from build123d import *

# Parameters (mm, degrees)
SKETCH_1_R          = 1.5
EXTRUDE_2_DEPTH     = 2
SKETCH_2_R          = 1.5
CUT_EXTRUDE_1_DEPTH = 10
SKETCH_3_R          = 0.5
CUT_EXTRUDE_2_DEPTH = 3
FILLET_1_R          = 1
SKETCH_4_R          = 0.5
SKETCH_4_W          = 24
SKETCH_4_H          = 6
CUT_EXTRUDE_3_DEPTH = 3


with BuildPart() as part:
    # 草图1 → 凸台-拉伸2 (new body)
    with BuildSketch(Plane.XY):
        with BuildLine():
            Line((56, -66.5), (44, -66.5))
            Line((44, -66.5), (44, -41.3))
            Line((44, -41.3), (56, -41.3))
            Line((56, -41.3), (56, -21.3))
            Line((56, -21.3), (44, -21.3))
            Line((44, -21.3), (44, -5.1))
            Line((44, -5.1), (56, -5.1))
            Line((56, -5.1), (56, 14.9))
            Line((56, 14.9), (44, 14.9))
            Line((44, 14.9), (44, 30.5))
            Line((44, 30.5), (56, 30.5))
            Line((56, 30.5), (56, 50.5))
            Line((56, 50.5), (44, 50.5))
            Line((44, 50.5), (44, 74.5))
            Line((44, 74.5), (0, 74.5))
            ThreePointArc((0, 74.5), (-23.145322016, 70.813445537), (-44, 60.118632719))
            Line((-44, 60.118632719), (-44, 40.5))
            Line((-44, 40.5), (-52, 40.5))
            Line((-52, 40.5), (-52, 20.5))
            Line((-52, 20.5), (-44, 20.5))
            Line((-44, 20.5), (-44, 0.5))
            Line((-44, 0.5), (-52, 0.5))
            Line((-52, 0.5), (-52, -19.5))
            Line((-52, -19.5), (-44, -19.5))
            Line((-44, -19.5), (-44, -44.5))
            Line((-44, -44.5), (-52, -44.5))
            Line((-52, -44.5), (-52, -59.5))
            Line((-52, -59.5), (-44, -59.5))
            Line((-44, -59.5), (-44, -64.5))
            Line((-44, -64.5), (-34, -74.5))
            Line((-34, -74.5), (-24, -74.5))
            Line((-24, -74.5), (-24, -92.324700538))
            Line((-24, -92.324700538), (-14.522169318, -97.796728634))
            Line((-14.522169318, -97.796728634), (-8, -86.5))
            Line((-8, -86.5), (-8, -74.5))
            Line((-8, -74.5), (19, -74.5))
            Line((19, -74.5), (19, -86.5))
            Line((19, -86.5), (56, -86.5))
            Line((56, -86.5), (56, -66.5))
        make_face()
        with Locations((24, -81.5)):
            Circle(SKETCH_1_R, mode=Mode.SUBTRACT)
        with Locations((39, -81.5)):
            Circle(SKETCH_1_R, mode=Mode.SUBTRACT)
        with Locations((51, -81.5)):
            Circle(SKETCH_1_R, mode=Mode.SUBTRACT)
        with Locations((16, 35.5)):
            Circle(SKETCH_1_R, mode=Mode.SUBTRACT)
        with Locations((39, 69.5)):
            Circle(SKETCH_1_R, mode=Mode.SUBTRACT)
        with Locations((39, -69.5)):
            Circle(SKETCH_1_R, mode=Mode.SUBTRACT)
        with Locations((-14, 35.5)):
            Circle(SKETCH_1_R, mode=Mode.SUBTRACT)
        with Locations((-16, -81.5)):
            Circle(SKETCH_1_R, mode=Mode.SUBTRACT)
        with Locations((-16, -91.17)):
            Circle(SKETCH_1_R, mode=Mode.SUBTRACT)
        with Locations((51, -35.5)):
            Circle(SKETCH_1_R, mode=Mode.SUBTRACT)
        with Locations((51, 4.5)):
            Circle(SKETCH_1_R, mode=Mode.SUBTRACT)
        with Locations((51, 35.5)):
            Circle(SKETCH_1_R, mode=Mode.SUBTRACT)
    extrude(amount=EXTRUDE_2_DEPTH)

    # 草图2 → 切除-拉伸1 (cut)
    with BuildSketch(Plane(origin=(0, 0, 0), x_dir=(-1, 0, 0), z_dir=(0, 0, -1))):
        with Locations((48.75, 30.5)):
            Circle(SKETCH_2_R)
        with Locations((48.75, -9.5)):
            Circle(SKETCH_2_R)
        with Locations((48.75, -52)):
            Circle(SKETCH_2_R)
    extrude(amount=-CUT_EXTRUDE_1_DEPTH, mode=Mode.SUBTRACT)

    # 草图3 → 切除-拉伸2 (cut, through all)
    with BuildSketch(Plane(origin=(0, 0, 0), x_dir=(-1, 0, 0), z_dir=(0, 0, -1))):
        with Locations((-44, 50.5)):
            Circle(SKETCH_3_R)
        with Locations((-44, 30.5)):
            Circle(SKETCH_3_R)
        with Locations((-44, 14.9)):
            Circle(SKETCH_3_R)
        with Locations((-44, -5.1)):
            Circle(SKETCH_3_R)
        with Locations((-44, -21.3)):
            Circle(SKETCH_3_R)
        with Locations((-44, -41.3)):
            Circle(SKETCH_3_R)
        with Locations((-44, -66.5)):
            Circle(SKETCH_3_R)
        with Locations((44, 40.5)):
            Circle(SKETCH_3_R)
        with Locations((44, 20.5)):
            Circle(SKETCH_3_R)
        with Locations((44, 0.5)):
            Circle(SKETCH_3_R)
        with Locations((44, -19.5)):
            Circle(SKETCH_3_R)
        with Locations((44, -44.5)):
            Circle(SKETCH_3_R)
        with Locations((44, -59.5)):
            Circle(SKETCH_3_R)
        with Locations((-19, -74.5)):
            Circle(SKETCH_3_R)
        with Locations((8, -74.5)):
            Circle(SKETCH_3_R)
        with Locations((24, -74.5)):
            Circle(SKETCH_3_R)
    extrude(amount=-CUT_EXTRUDE_2_DEPTH, mode=Mode.SUBTRACT)

    # 圆角1
    fillet_1_edges = [part.edges().sort_by_distance(p)[0] for p in [
        (-8, -86.5, 1),
        (-14.522169318, -97.796728634, 1),
        (-24, -92.324700538, 1),
        (-34, -74.5, 1),
        (-44, -64.5, 1),
        (-52, -59.5, 1),
        (-52, -44.5, 1),
        (-52, -19.5, 1),
        (-52, 0.5, 1),
        (-52, 20.5, 1),
        (-52, 40.5, 1),
        (-44, 60.118632719, 1),
        (44, 74.5, 1),
        (56, 50.5, 1),
        (56, 30.5, 1),
        (56, -5.1, 1),
        (56, -21.3, 1),
        (56, -41.3, 1),
        (56, -66.5, 1),
        (56, -86.5, 1),
        (19, -86.5, 1),
    ]]
    fillet(fillet_1_edges, radius=FILLET_1_R)

    # 草图4 → 切除-拉伸3 (cut, through all)
    with BuildSketch(Plane(origin=(0, 0, 0), x_dir=(-1, 0, 0), z_dir=(0, 0, -1))):
        with BuildLine():
            Line((-12, 64), (-12, 64.5))
            Line((-12, 64.5), (-11.5, 64.5))
            ThreePointArc((-11.5, 64.5), (-12.353553391, 64.853553391), (-12, 64))
        make_face()
        with BuildLine():
            Line((-11.5, 64.5), (-12, 64.5))
            Line((-12, 64.5), (-12, 64))
            ThreePointArc((-12, 64), (-11.646446609, 64.146446609), (-11.5, 64.5))
        make_face()
        with BuildLine():
            ThreePointArc((-11.5, 58.5), (-11.646446609, 58.853553391), (-12, 59))
            Line((-12, 59), (-12, 58.5))
            Line((-12, 58.5), (-11.5, 58.5))
        make_face()
        with BuildLine():
            Line((-12, 58.5), (-12, 59))
            ThreePointArc((-12, 59), (-12.353553391, 58.146446609), (-11.5, 58.5))
            Line((-11.5, 58.5), (-12, 58.5))
        make_face()
        with Locations((12, 58.5)):
            Circle(SKETCH_4_R)
        with Locations((12, 64.5)):
            Circle(SKETCH_4_R)
        with Locations((-12, 64.5)):
            Circle(SKETCH_4_R)
        with Locations((-12, 58.5)):
            Circle(SKETCH_4_R)
        with Locations((0, 61.5)):
            Rectangle(SKETCH_4_W, SKETCH_4_H)
        with BuildLine():
            ThreePointArc((12.5, 64.5), (12, 65), (11.5, 64.5))
            Line((11.5, 64.5), (12, 64.5))
            Line((12, 64.5), (12, 64))
            ThreePointArc((12, 64), (12.353553391, 64.146446609), (12.5, 64.5))
        make_face()
        with BuildLine():
            Line((12, 64.5), (11.5, 64.5))
            ThreePointArc((11.5, 64.5), (11.646446609, 64.146446609), (12, 64))
            Line((12, 64), (12, 64.5))
        make_face()
        with BuildLine():
            ThreePointArc((12.5, 58.5), (12.353553391, 58.853553391), (12, 59))
            Line((12, 59), (12, 58.5))
            Line((12, 58.5), (11.5, 58.5))
            ThreePointArc((11.5, 58.5), (12, 58), (12.5, 58.5))
        make_face()
        with BuildLine():
            Line((12, 58.5), (12, 59))
            ThreePointArc((12, 59), (11.646446609, 58.853553391), (11.5, 58.5))
            Line((11.5, 58.5), (12, 58.5))
        make_face()
    extrude(amount=-CUT_EXTRUDE_3_DEPTH, mode=Mode.SUBTRACT)


solid = part.part
Input: part model. Units: mm. Frame: model coordinates. Round coordinates to 2 decimals unless told otherwise and drop trailing zeros. Write each loop counter-clockwise with the first axis right and the second up, starting at its lowest first coordinate (ties: lowest second). Pieces come first, ordered by that corner, then holes.
1) Cut plane B-B (y = -27.5). Return the cut outline in (x, z), then the cut area to 3 significant figures.
2) Cut plane A-A (z = 1.2). Count the separate pieces of the cut face and the enclosed holes in it, then the cut area to 3 significant figures.
3) Ray query, L1, parallel to Y at x = 2.5, z = 1.55; L2, parallel to X at y = 34.5, z = 0.65; L3, parallel to X at y = 9.5, z = 0.8. Return the intervals inside material, ascending.
4) Contact query for flat-ended pins moving along their axis: P1, Ø1, axis at x = -9, z = 0.5, coming from the +Y side; P2, Ø1, axis at y = -57, z = 1, coming from the +X side; P3, Ø0.6, axis at y = -29, z = 0.5, coming from the -X side; P4, Ø1.8, axis at x = -48.75, y = -9.5, coming from the -Z side. Output: stop coordinate, or through.
5) Cut plane C-C (x = -27). Return the cut outline in (y, z), then the cut area to 3 significant figures.
Geometry says:
1. outline: (-44, 0) - (56, 0) - (56, 2) - (-44, 2) - close
1. area: 200 mm2
2. separate pieces: 1
2. enclosed holes: 16
2. area: 14,600 mm2
3. L1: y = -74.5 to 58.5, 64.5 to 74.5
3. L2: x = -52 to -15.12, -12.88 to 14.88, 17.12 to 49.88, 52.12 to 56
3. L3: x = -44 to 56
4. P1: stops at y = 74.01
4. P2: stops at x = 44
4. P3: stops at x = -44
4. P4: passes through
5. outline: (-74.5, 0) - (69.44, 0) - (69.44, 2) - (-74.5, 2) - close
5. area: 288 mm2
